Work out the finished part from the listing and answer in its coordinate system (mm). Face numbers are marked on the shaded views. Give positions to 0.01 mm unless a question says otherwise; leave off trailing zeros. Order: outer loops, then holes, each group sorted by start corner. A loop starts at its lowest first (then second) coordinate and runs counter-clockwise, first axis right, second up. Notation, with made-up numbers: M 36,15.25 L 85,15.25 A27 cw 85,40.25 Z; hole C 59.5,-12.5 d11. An arc over 180 degrees is marked long. One line per item, written item: value.
from build123d import *

# Parameters (mm, degrees)
F1_DEPTH = 5
F2_T     = -2.5
F4_DEPTH = 5.001
F5_R     = 2
F6_DEPTH = 5.001
F7_R     = 4
F7_R_2   = 2
F8_DEPTH = 2.5


with BuildPart() as f1:
    # F0 (on Front) → F1 (new body)
    with BuildSketch(Plane.XZ):
        Polygon((0, 95.369), (0, 0), (100.232048, 0), (100.232048, 37.5), align=None)
    extrude(amount=F1_DEPTH)

    # F2
    f2_openings = [f1.faces().sort_by_distance(p)[0] for p in [
        (42.840276, 0, 35.317578),
    ]]
    offset(amount=F2_T, openings=f2_openings)

    # F3 (on face) → F4 (cut, through all)
    with BuildSketch(Plane(origin=(0, 0, 0), x_dir=(-1, 0, 0), z_dir=(0, 1, 0))):
        Polygon((-90.232048, 37.5), (-95.232048, 34.613249), (-95.232048, 5), (-90.232048, 5), align=None)
        Polygon((-85.232048, 40.386751), (-85.232048, 5), (-80.232048, 5), (-80.232048, 43.273503), align=None)
        Polygon((-75.232048, 46.160254), (-75.232048, 5), (-70.232048, 5), (-70.232048, 49.047005), align=None)
        Polygon((-65.232048, 51.933757), (-65.232048, 5), (-60.232048, 5), (-60.232048, 54.820508), align=None)
        Polygon((-55.232048, 57.707259), (-55.232048, 5), (-50.232048, 5), (-50.232048, 60.594011), align=None)
        Polygon((-50.232048, 60.594011), (-50.232048, 5), (-45.232048, 5), (-45.232048, 63.480762), align=None)
        Polygon((-45.232048, 63.480762), (-45.232048, 5), (-40.232048, 5), (-40.232048, 66.367513), align=None)
        Polygon((-30.232048, 72.141016), (-35.232048, 69.254265), (-35.232048, 5), (-30.232048, 5), align=None)
        Polygon((-25.232048, 75.027767), (-30.232048, 72.141016), (-30.232048, 5), (-25.232048, 5), align=None)
        Polygon((-20.232048, 77.914519), (-25.232048, 75.027767), (-25.232048, 5), (-20.232048, 5), align=None)
    extrude(amount=-F4_DEPTH, mode=Mode.SUBTRACT)

    # F5 (on face) → F6 (cut, through all)
    with BuildSketch(Plane(origin=(0, 0, 0), x_dir=(-1, 0, 0), z_dir=(0, 1, 0))):
        with Locations((-12.5, 60)):
            Circle(F5_R)
        with Locations((-12.5, 20)):
            Circle(F5_R)
    extrude(amount=-F6_DEPTH, mode=Mode.SUBTRACT)

    # F7 (on face) → F8 (join, through all)
    with BuildSketch(Plane(origin=(0, -2.5, 0), x_dir=(-1, 0, 0), z_dir=(0, 1, 0))):
        with Locations((-12.5, 60)):
            Circle(F7_R)
        with Locations((-12.5, 60)):
            Circle(F7_R_2, mode=Mode.SUBTRACT)
        with Locations((-12.5, 20)):
            Circle(F7_R)
        with Locations((-12.5, 20)):
            Circle(F7_R_2, mode=Mode.SUBTRACT)
    extrude(amount=F8_DEPTH)


solid = f1.part
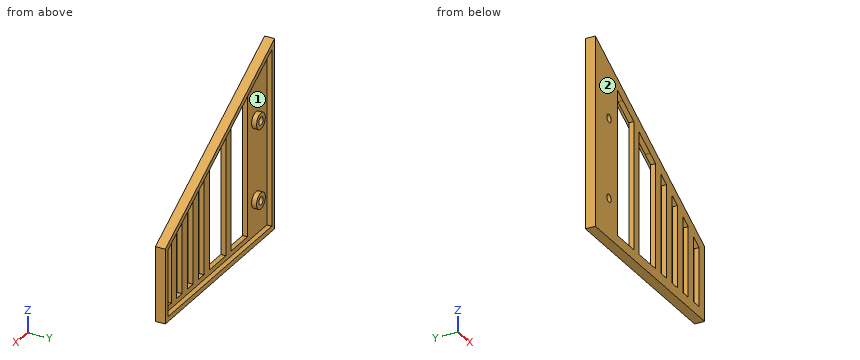
(1) Section D-D, the plane x = 63 is taken. Give the vertices of the cut face in (y, z), then the cut area to 3 significant figures.
Findings:
outline: M -5,0 L 0,0 L 0,2.5 L -2.5,2.5 L -2.5,5 L -5,5 Z; M -5,53.22 L -2.5,53.22 L -2.5,56.11 L 0,56.11 L 0,59 L -5,59 Z
area: 40.4 mm^2
(2) Given P1, Ø3, axis at x = 82, y = -4, coming from the +Z side; P2, Ø1.2, axis at x = 93.5, y = -3.5, coming from the +Z side; P3, Ø3.5, axis at x = 12.5, z = 60, coming from the -Y side (3 decimals); P4, Ø3, axis at x = 64, y = -1.5, coming from the +Z side, each flat-ended and moving along its own axis, determine where each tip first touches the part or whether it passes through.
Findings:
P1: stops at z = 48.89
P2: stops at z = 41.73
P3: passes through
P4: stops at z = 59.28
(3) Determine the mould class of the marked faces 1 and 2 for opening direction Z: pulls with the +Z half, pulls with the -Z half, needs draft (parallel to the pull), parting line crosses it, or undercut.
Findings:
face 1: undercut
face 2: needs draft
(4) Section A-A, the plane y = -1.75 is taken. Give the vertices of the cut face in (x, z).
Findings:
outline: M 0,0 L 100.23,0 L 100.23,37.5 L 0,95.37 Z; C 12.5,20 d8; C 12.5,60 d8; hole M 2.5,2.5 L 97.73,2.5 L 97.73,36.06 L 2.5,91.04 Z; hole C 12.5,20 d4; hole C 12.5,60 d4
(5) Section B-B, the plane x = 12.5 is taken. Give the vertices of the cut face in (y, z), then the cut area to 3 significant figures.
Findings:
outline: M -5,0 L 0,0 L 0,2.5 L -2.5,2.5 L -2.5,16 L 0,16 L 0,18 L -5,18 Z; M -5,22 L 0,22 L 0,24 L -2.5,24 L -2.5,56 L 0,56 L 0,58 L -5,58 Z; M -5,62 L 0,62 L 0,64 L -2.5,64 L -2.5,85.27 L 0,85.27 L 0,88.15 L -5,88.15 Z
area: 234 mm^2
(6) Section C-C, the plane z = 20 is taken. Give the number of separate pieces and of enclosed holes in the cut face, then the cut area to 3 significant figures.
Findings:
separate pieces: 8
enclosed holes: 0
area: 138 mm^2
(7) Find the intervals of material crossed by probe 1 along Z at (x, y) = (9, -1.7); probe 2 along Z at (x, y) = (12.5, -4.15); probe 3 along X at (y, z) = (-4.4, 49.5), in increasing order. Write a range as from..to.
Findings:
probe 1: z = 0..2.5, 18.06..21.94, 58.06..61.94, 87.29..90.17
probe 2: z = 0..18, 22..58, 62..88.15
probe 3: x = 0..20.23, 35.23..40.23, 55.23..60.23, 65.23..79.45
